from build123d import *

# Parameters (mm, degrees)
RESSALTO_EXTRUS_O1_DEPTH      = 5
RESSALTO_EXTRUS_O1_DEPTH_BACK = 5
CORTE_EXTRUS_O1_DEPTH         = 5
CORTE_EXTRUS_O1_DEPTH_BACK    = 5
ESBO_O2_R                     = 4
ESBO_O3_R                     = 2.5
CORTE_EXTRUS_O2_DEPTH         = 30.580398915


with BuildPart() as part:
    # Esbo_o1 → Ressalto-extrus_o1 (new, two sides: drawn at the far end of the back side and taken through both)
    with BuildSketch(Plane(origin=(0, 0, 0), x_dir=(1, 0, 0), z_dir=(0, 1, 0)).offset(-RESSALTO_EXTRUS_O1_DEPTH_BACK)):
        with BuildLine():
            Line((-15, 0), (-15, -10))
            Line((-15, -10), (-25, -10))
            Line((-25, -10), (-25, -15))
            Line((-25, -15), (25, -15))
            Line((25, -15), (25, -10))
            Line((25, -10), (15, -10))
            Line((15, -10), (15, 0))
            ThreePointArc((15, 0), (0, 15), (-15, 0))
        make_face()
    extrude(amount=RESSALTO_EXTRUS_O1_DEPTH + RESSALTO_EXTRUS_O1_DEPTH_BACK)

    # Esbo_o2 → Corte-extrus_o1 (cut, two sides: drawn at the far end of the back side and taken through both)
    with BuildSketch(Plane(origin=(0, 0, 0), x_dir=(1, 0, 0), z_dir=(0, 1, 0)).offset(-CORTE_EXTRUS_O1_DEPTH_BACK)):
        with Locations(Location((0, 0, 0), (0, 0, 270))):
            Circle(ESBO_O2_R)
    extrude(amount=CORTE_EXTRUS_O1_DEPTH + CORTE_EXTRUS_O1_DEPTH_BACK, mode=Mode.SUBTRACT)

    # Esbo_o3 → Corte-extrus_o2 (cut, through all)
    with BuildSketch(Plane.XY):
        with Locations(Location((21.5, 0, 0), (0, 0, 180))):
            Circle(ESBO_O3_R)
        with Locations(Location((-21.5, 0, 0), (0, 0, 180))):
            Circle(ESBO_O3_R)
    extrude(amount=CORTE_EXTRUS_O2_DEPTH, mode=Mode.SUBTRACT)


solid = part.part
CAD build for the part. Positions are in the model's coordinates, mm. A direction names the side the tool comes from. Round coordinates to 2 decimals unless told otherwise and drop trailing zeros. Write each loop counter-clockwise with the first axis right and the second up, starting at its lowest first coordinate (ties: lowest second). Pieces come first, ordered by that corner, then holes. Notation, with made-up numbers: M -15,84 L -4,84 A19 ccw -4,109 Z; hole C 36.5,33.25 d9. An arc over 180 degrees is marked long. Put each result on its own line as item: value. Start each with the question number.
1) Saw through at D-D, the plane z = -2.75. Write the cut outline in (x, y), and give its area (3 significant figures).
2) Saw through at C-C, the plane y = -4. Write the cut outline in (x, z).
3) Pin check, flat tips, straight feed: pin 1 Ø5 at (y, z) = (3, 7) entering from -X; pin 2 Ø4 at (y, z) = (0, -10) entering from +X; pin 3 Ø1.5 at (y, z) = (0, -9) entering from +X; pin 4 Ø6 at (x, y) = (21.5, 0) entering from +Z. Stop position of each tip, or through.
4) Saw through at A-A, the plane y = 0. Write the cut outline in (x, z).
5) Saw through at B-B, the plane x = -21.5. Write the cut outline in (y, z), and give its area (3 significant figures).
6) Pull direction X, two halves, no side cores. Call faces 4 (the cylindrical face through (24, 0, 12)), 5 (the flat face through (19, 1, 10)), 6 (the cylindrical face through (0, 0, -15)), 7 (the flat face through (-25, 0, 12)): pulls with the +X half, pulls with the -X half, needs draft (parallel to the pull), parting line crosses it, or undercut.
7) 3-axis set-ups, long thin cutter, end or side, ignore diameter. For faces 1 (the flat face through (15, 0, 5)), 2 (the flat face through (25, 0, 13)), 3 (the flat face through (-18.8, -0.1, 10)): which of +Z, -Z, +X, -X, +Y, -Y reach the whole face in a straight line?
8) Drill centre lines: probe 1 along Y at (x, z) = (-21.5, 12.9); probe 2 along X at (y, z) = (4, 2.75); probe 3 along Z at (x, y) = (18.5, -0.75). Where is each one in solid material? Low to high. Write a range as [from, to].
Resolved:
1. outline: M -14.75,-5 L -2.9,-5 L -2.9,5 L -14.75,5 Z; M 2.9,-5 L 14.75,-5 L 14.75,5 L 2.9,5 Z
1. area: 237 mm²
2. outline: M -25,10 L -15,10 L -15,0 A15 ccw 15,0 L 15,10 L 25,10 L 25,15 L -25,15 Z; hole C 0,0 d8
3. pin 1: x = -15
3. pin 2: x = 12.69
3. pin 3: x = 12.53
3. pin 4: z = 15
4. outline: M -25,10 L -24,10 L -24,15 L -25,15 Z; M -19,10 L -15,10 L -15,0 A15 ccw 15,0 L 15,10 L 19,10 L 19,15 L -19,15 Z; M 24,10 L 25,10 L 25,15 L 24,15 Z; hole C 0,0 d8
5. outline: M -5,10 L -2.5,10 L -2.5,15 L -5,15 Z; M 2.5,10 L 5,10 L 5,15 L 2.5,15 Z
5. area: 25.0 mm²
6. face 4: undercut
6. face 5: needs draft
6. face 6: parting line crosses it
6. face 7: pulls with the -X half
7. face 1: -Z, +X, +Y, -Y
7. face 2: +Z, -Z, +X, +Y, -Y
7. face 3: -Z, -X, +Y, -Y
8. probe 1: [-5, -2.5], [2.5, 5]
8. probe 2: [-15, -2.9], [2.9, 15]
8. probe 3: [10, 15]
